from build123d import *

# Parameters (mm, degrees)
SKETCH1_W                    = 64
SKETCH1_H                    = 178.8
BASE_FLANGE1_DEPTH           = 1.6
EDGE_FLANGE1_STRIP_W         = 9.6
EDGE_FLANGE1_STRIP_H         = 1.6
EDGE_FLANGE1_STRIP_CUT_DEPTH = 64
EDGE_FLANGE1_DEPTH           = 64
EDGE_FLANGE2_STRIP_W         = 9.6
EDGE_FLANGE2_STRIP_H         = 1.6
EDGE_FLANGE2_STRIP_CUT_DEPTH = 64
EDGE_FLANGE2_DEPTH           = 64
SKETCH12_R                   = 2.1
CUT_EXTRUDE1_DEPTH           = 1000
SKETCH13_R                   = 1.75
SKETCH13_R_2                 = 2
CUT_EXTRUDE2_DEPTH           = 1000
SKETCH14_R                   = 3.5
CUT_EXTRUDE3_DEPTH           = 5
SKETCH15_W                   = 4.498408697
SKETCH15_H                   = 14.372964376
CUT_EXTRUDE4_DEPTH           = 10


# Sheet-metal steps are written as plain solids
with BuildPart() as part:
    # Sketch1 → Base-Flange1 (new body)
    with BuildSketch(Plane.XY):
        with Locations((32, 89.4)):
            Rectangle(SKETCH1_W, SKETCH1_H)
    extrude(amount=-BASE_FLANGE1_DEPTH)

    # Edge-Flange1 strip (across the edge) → Edge-Flange1 strip cut (cut)
    with BuildSketch(Plane(origin=(64, 0, -1.6), x_dir=(0, 1, 0), z_dir=(-1, 0, 0))):
        with Locations((-1.6, -0.8)):
            Rectangle(EDGE_FLANGE1_STRIP_W, EDGE_FLANGE1_STRIP_H)
    extrude(amount=EDGE_FLANGE1_STRIP_CUT_DEPTH, mode=Mode.SUBTRACT)

    # Edge-Flange1 section (across the edge) → Edge-Flange1 (add)
    with BuildSketch(Plane(origin=(64, 0, -1.6), x_dir=(0, 1, 0), z_dir=(-1, 0, 0))):
        with BuildLine():
            Line((0, 1.6), (0, 12.4))
            Line((0, 12.4), (1.6, 12.4))
            Line((1.6, 12.4), (1.6, 1.6))
            ThreePointArc((1.6, 1.6), (2.06862915, 0.46862915), (3.2, 0))
            Line((3.2, 0), (3.2, -1.6))
            ThreePointArc((3.2, -1.6), (0.9372583, -0.6627417), (0, 1.6))
        make_face()
    extrude(amount=EDGE_FLANGE1_DEPTH)

    # Edge-Flange2 strip (across the edge) → Edge-Flange2 strip cut (cut)
    with BuildSketch(Plane(origin=(0, 178.8, -1.6), x_dir=(0, -1, 0), z_dir=(1, 0, 0))):
        with Locations((-1.6, -0.8)):
            Rectangle(EDGE_FLANGE2_STRIP_W, EDGE_FLANGE2_STRIP_H)
    extrude(amount=EDGE_FLANGE2_STRIP_CUT_DEPTH, mode=Mode.SUBTRACT)

    # Edge-Flange2 section (across the edge) → Edge-Flange2 (add)
    with BuildSketch(Plane(origin=(0, 178.8, -1.6), x_dir=(0, -1, 0), z_dir=(1, 0, 0))):
        with BuildLine():
            Line((0, 1.6), (0, 12.4))
            Line((0, 12.4), (1.6, 12.4))
            Line((1.6, 12.4), (1.6, 1.6))
            ThreePointArc((1.6, 1.6), (2.06862915, 0.46862915), (3.2, 0))
            Line((3.2, 0), (3.2, -1.6))
            ThreePointArc((3.2, -1.6), (0.9372583, -0.6627417), (0, 1.6))
        make_face()
    extrude(amount=EDGE_FLANGE2_DEPTH)

    # Sketch12 → Cut-Extrude1 (cut)
    with BuildSketch(Plane.XZ):
        with Locations(Location((45.791182174, -8, 0), (0, 0, 270))):
            Circle(SKETCH12_R)
        with Locations(Location((13.491811911, -8, 0), (0, 0, 270))):
            Circle(SKETCH12_R)
    extrude(amount=-CUT_EXTRUDE1_DEPTH, mode=Mode.SUBTRACT)

    # Sketch13 → Cut-Extrude2 (cut)
    with BuildSketch(Plane.XY):
        with Locations((61.291182174, 16)):
            Circle(SKETCH13_R)
        with Locations((29.639685291, 40.768563608)):
            Circle(SKETCH13_R_2)
        with Locations((42.339685291, 53.468563608)):
            Circle(SKETCH13_R_2)
        with Locations((16.939685291, 53.468563608)):
            Circle(SKETCH13_R_2)
        with Locations((29.639685291, 66.168563608)):
            Circle(SKETCH13_R_2)
    extrude(amount=-CUT_EXTRUDE2_DEPTH, mode=Mode.SUBTRACT)

    # Sketch14 → Cut-Extrude3 (cut)
    with BuildSketch(Plane.XY):
        with Locations((29.384576347, 53.812205541)):
            Circle(SKETCH14_R)
    extrude(amount=-CUT_EXTRUDE3_DEPTH, mode=Mode.SUBTRACT)

    # Sketch15 → Cut-Extrude4 (cut)
    with BuildSketch(Plane.XY):
        with Locations((50.891201279, 13.989760377)):
            Rectangle(SKETCH15_W, SKETCH15_H)
    extrude(amount=-CUT_EXTRUDE4_DEPTH, mode=Mode.SUBTRACT)


solid = part.part
Work out the finished part from the listing and answer in its coordinate system (mm). A direction names the side the tool comes from. Coordinates: 2 decimals unless noted, no trailing zeros. Write each loop counter-clockwise with the first axis right and the second up, starting at its lowest first coordinate (ties: lowest second). Pieces come first, ordered by that corner, then holes.
1. The part is cut by section D-D, the plane y = 130. Write down the section's boundary in (x, z).
Results list:
outline: (0, -1.6) - (64, -1.6) - (64, 0) - (0, 0) - close
2. For a pull along Z with two mould halves and no side action, classify faces 3 (the cylindrical face through (32.448, 0.962, -0.913)), 4 (the cylindrical face through (43.741, 0.789, -7.545)), 5 (the cylindrical face through (15.574, 0.789, -7.727)), 6 (the flat face through (0, 89, -1)) as +Z half, -Z half, draft (parallel to the pull), parting line (faces both ways), or undercut.
Results list:
face 3: +Z half
face 4: undercut
face 5: undercut
face 6: draft
3. The part is cut by section A-A, the plane y = 16. Write down the section's boundary in (x, z), and give its area (3 significant figures).
Results list:
outline: (0, -1.6) - (48.64, -1.6) - (48.64, 0) - (0, 0) - close; (53.14, -1.6) - (59.54, -1.6) - (59.54, 0) - (53.14, 0) - close; (63.04, -1.6) - (64, -1.6) - (64, 0) - (63.04, 0) - close
area: 89.6 mm2
4. Flat-ended cylindrical pins translate along their axes: pin 1 (0.8 mm diameter, centred on y = 16.5, z = -1, fed in from -X); pin 2 (6 mm diameter, centred on x = 10, y = 38, fed in from -Z); pin 3 (0.5 mm diameter, centred on x = 50.5, z = -0.5, fed in from +Y); pin 4 (4 mm diameter, centred on x = 45.79, z = -8, fed in from +Y). Find the tip coordinate at first contact, or state that the pin passes through.
Results list:
pin 1: stops at x = 0
pin 2: stops at z = -1.6
pin 3: stops at y = 177.66
pin 4: passes through
5. The part is cut by section B-B, the plane z = -8. Write down the section's boundary in (x, y), and give its area (3 significant figures).
Results list:
outline: (0, 0) - (11.39, 0) - (11.39, 1.6) - (0, 1.6) - close; (0, 177.2) - (11.39, 177.2) - (11.39, 178.8) - (0, 178.8) - close; (15.59, 0) - (43.69, 0) - (43.69, 1.6) - (15.59, 1.6) - close; (15.59, 177.2) - (43.69, 177.2) - (43.69, 178.8) - (15.59, 178.8) - close; (47.89, 0) - (64, 0) - (64, 1.6) - (47.89, 1.6) - close; (47.89, 177.2) - (64, 177.2) - (64, 178.8) - (47.89, 178.8) - close
area: 178 mm2
6. For faces 1 (the flat face through (64, 89, -1)), 2 (the flat face through (32, 91, -1.6)), determine the directions among +Z, -Z, +X, -X, +Y, -Y from which every point of the face is accessible in a straight line to the end or side of a thin tool.
Results list:
face 1: +Z, -Z, +X, +Y, -Y
face 2: -Z, +X, -X
7. Consider line 1 along Y through (x, z) = (17, -7.25); line 2 along Z through (x, y) = (38.5, 55.5). Determine where each line is inside the solid, lowest interval first.
Results list:
line 1: y = 0 to 1.6, 177.2 to 178.8
line 2: z = -1.6 to 0
8. The part is cut by section C-C, the plane x = 21. Write down the section's boundary in (y, z), and give its area (3 significant figures).
Results list:
outline: (0, -14) - (1.6, -14) - (1.6, -3.2) arc R1.6 cw to (3.2, -1.6) - (175.6, -1.6) arc R1.6 cw to (177.2, -3.2) - (177.2, -14) - (178.8, -14) - (178.8, -3.2) arc R3.2 ccw to (175.6, 0) - (3.2, 0) arc R3.2 ccw to (0, -3.2) - close
area: 322 mm2
